For this review, take the finished solid that the model builds, in its own axes (mm). Coordinates: 2 decimals unless noted, no trailing zeros. Write each loop counter-clockwise with the first axis right and the second up, starting at its lowest first coordinate (ties: lowest second). Pieces come first, ordered by that corner, then holes. Notation, with made-up numbers: (-23.5, 3.25) -> (19.5, 3.25) arc R17 cw to (19.5, 35.25) -> close; hole circle Ø2 at (72, -28). An arc over 180 degrees is marked (long way). Put each result on its own line as item: value. Start each with the question number.
Item 1: Insertion check: P1, Ø2.5, axis at x = 23.5, y = 3, coming from the +Z side. The pin has a flat end and moves straight along its axis. Give the tip position at first contact, or say it passes through.
Item 2: Consider section C-C on x = 13. Give the boundary of the cut face in (y, z).
Item 3: Consider section A-A on y = 3. Give the boundary of the cut face in (x, z).
Item 4: Consider section B-B on z = 0.3. Give the boundary of the cut face in (x, y), and give its area (3 significant figures).
Item 5: Consider section D-D on y = 22. Give the boundary of the cut face in (x, z), and give its area (3 significant figures).
Item 6: The part is to be moulded in two halves that separate along X. For faces 1 (the cylindrical face through (3.676, 32.692, 0.76)), 2 (the cylindrical face through (2.68, 23.17, 0.74)), 3 (the flat face through (13, -4, 1)), say which applies: +X half, -X half, draft (parallel to the pull), parting line (faces both ways), or undercut.
Item 7: To check wall thickness, follow L1, parallel to Y at x = 22.75, z = 0.3; L2, parallel to Y at x = 13, z = 1.1; L3, parallel to Y at x = 2.5, z = 0.45. State the ranges of each line that lie inside material, in increasing order.
Autodesk Inventor part; units mm, degrees
ref_plane "YZ Plane" through (0, 0, 0) normal (1, 0, 0) x (0, 1, 0)
ref_plane "XZ Plane" through (0, 0, 0) normal (0, 1, 0) x (-1, 0, 0)
ref_plane "XY Plane" through (0, 0, 0) normal (0, 0, 1) x (1, 0, 0)
sketch "スケッチ2" plane through (0, 0, 0) normal (0, 0, 1) x (1, 0, 0)
  line L0 (0, 0) -> (26, 0)
  line L1 (26, 0) -> (26, 33)
  line L2 (26, 33) -> (0, 33)
  line L3 (0, 33) -> (0, 0)
  line L4 (0, 0) -> (26, 0)
  line L5 (26, 0) -> (26, 24)
  line L6 (26, 24) -> (0, 24) construction
  line L7 (0, 24) -> (0, 0)
  circle A0 centre (13, 24) radius 13
  circle A1 centre (13, 24) radius 6.25
  line L8 (26, 0) -> (0, 0)
  line L9 (0, 0) -> (0, -4)
  line L10 (0, -4) -> (26, -4)
  line L11 (26, -4) -> (26, 0)
  circle A2 centre (21, -2) radius 0.8
  circle A3 centre (5, -2) radius 0.8
  point P0 (22.3808, 33)
  point P1 (3.6192, 33)
  point P2 (26, -2)
  dimension "d0" = 26
  dimension "d1" = 33
  dimension "d2" = 24
  dimension "d3" = 12.5
  dimension "d8" = 4
  dimension "d9" = 1.6
  dimension "d10" = 1.6
  dimension "d12" = 5
  dimension "d13" = 5
extrude "押し出し1" add sketch "スケッチ2" along normal blind 1.5 contours L3 A0 L1 L0 | L0 L11 L10 L9 | A0 L2 picked at (12.7489, 32.0681)
sketch "スケッチ3" plane through (0, 0, 0) normal (0, 0, -1) x (-1, 0, 0)
  circle A0 centre (-2.5, 24) radius 0.85
  circle A1 centre (-23.5, 24) radius 0.85
  circle A2 centre (-23.5, 3) radius 0.85
  circle A3 centre (-2.5, 3) radius 0.85
  point P0 (0, 0)
extrude "押し出し2" cut sketch "スケッチ3" against normal through all
fillet "フィレット1" radius 3 4 edges at (22.3808, 33, 0.75) (3.6192, 33, 0.75) (26, -4, 0.75) (0, -4, 0.75)
equation "\"d13\" = d12"
equation "\"BendRadius\" = Thickness"
equation "\"BendReliefWidth\" = Thickness"
equation "\"BendReliefDepth\" = 0.5 * Thickness"
equation "\"CornerReliefSize\" = 4 * Thickness"
equation "\"MinimumRemnant\" = 2 * Thickness"
equation "\"TransitionRadius\" = BendRadius"
equation "\"JacobiRadiusSize\" = BendRadius"
equation "\"GapSize\" = Thickness"
properties part number "arm" material "アルミニウム 6061"
Return value:
1. P1: z = 1.5
2. outline: (-4, 0) -> (17.75, 0) -> (17.75, 1.5) -> (-4, 1.5) -> close; (30.25, 0) -> (33, 0) -> (33, 1.5) -> (30.25, 1.5) -> close
3. outline: (0, 0) -> (1.65, 0) -> (1.65, 1.5) -> (0, 1.5) -> close; (3.35, 0) -> (22.65, 0) -> (22.65, 1.5) -> (3.35, 1.5) -> close; (24.35, 0) -> (26, 0) -> (26, 1.5) -> (24.35, 1.5) -> close
4. outline: (0, -1) arc R3 ccw to (3, -4) -> (23, -4) arc R3 ccw to (26, -1) -> (26, 24) arc R13 ccw to (23.4, 31.8) arc R3 ccw to (21, 33) -> (5, 33) arc R3 ccw to (2.6, 31.8) arc R13 ccw to (0, 24) -> close; hole circle Ø1.7 at (2.5, 3); hole circle Ø1.7 at (2.5, 24); hole circle Ø1.6 at (5, -2); hole circle Ø12.5 at (13, 24); hole circle Ø1.6 at (21, -2); hole circle Ø1.7 at (23.5, 3); hole circle Ø1.7 at (23.5, 24)
4. area: 801 mm^2
5. outline: (0, 0) -> (7.08, 0) -> (7.08, 1.5) -> (0, 1.5) -> close; (18.92, 0) -> (26, 0) -> (26, 1.5) -> (18.92, 1.5) -> close
5. area: 21.2 mm^2
6. face 1: -X half
6. face 2: undercut
6. face 3: draft
7. L1: -4 to 2.6, 3.4 to 23.6, 24.4 to 32.44
7. L2: -4 to 17.75, 30.25 to 33
7. L3: -3.96 to 2.15, 3.85 to 23.15, 24.85 to 31.66
